Design review of the part built by this model. Coordinates are the model's own, in mm. Face numbers are marked on the shaded views. A direction names the side the tool comes from. Give positions to 0.01 mm unless a question says otherwise; leave off trailing zeros. Write each loop counter-clockwise with the first axis right and the second up, starting at its lowest first coordinate (ties: lowest second). Pieces come first, ordered by that corner, then holes. Notation, with made-up numbers: M -19,-30.75 L 39,-30.75 A20 cw 39,-1.75 Z; hole C 88,7.5 d5. An arc over 180 degrees is marked long. Answer in a Markdown table with one row per item.
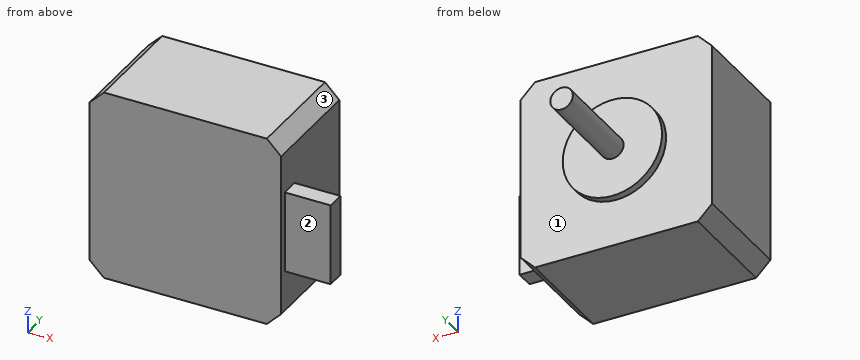
Autodesk Inventor part; units mm, degrees
ref_plane "YZ Plane" through (0, 0, 0) normal (1, 0, 0) x (0, 1, 0)
ref_plane "XZ Plane" through (0, 0, 0) normal (0, 1, 0) x (-1, 0, 0)
ref_plane "XY Plane" through (0, 0, 0) normal (0, 0, 1) x (1, 0, 0)
sketch "Sketch1" plane through (0, 0, 0) normal (0, 1, 0) x (-1, 0, 0)
  line L0 (-18.034, 21.209) -> (18.034, 21.209)
  line L1 (21.209, 18.034) -> (21.209, -18.034)
  line L2 (18.034, -21.209) -> (-18.034, -21.209)
  line L3 (-21.209, -18.034) -> (-21.209, 18.034)
  line L4 (-21.209, 21.209) -> (21.209, -21.209) construction
  line L5 (21.209, 21.209) -> (-21.209, -21.209) construction
  line L6 (21.209, 18.034) -> (18.034, 21.209)
  line L7 (18.034, -21.209) -> (21.209, -18.034)
  line L8 (-18.034, -21.209) -> (-21.209, -18.034)
  line L9 (-21.209, 18.034) -> (-18.034, 21.209)
  point P0 (0, 0)
  dimension "d0" = 42.418
  dimension "d1" = 3.175
  dimension "d2" = 3.175
  dimension "d3" = 3.175
  dimension "d4" = 3.175
  dimension "d5" = 3.175
  dimension "d6" = 3.175
  dimension "d7" = 3.175
  dimension "d8" = 3.175
extrude "Extrusion1" add sketch "Sketch1" along normal blind 23.876
sketch "Sketch2" plane through (0, 23.876, 0) normal (0, 1, 0) x (1, 0, 0)
  circle A0 centre (0, 0) radius 10.9982
  dimension "d11" = 21.9964
extrude "Extrusion2" add sketch "Sketch2" along normal blind 1.651
sketch "Sketch3" plane through (0, 25.527, 0) normal (0, 1, 0) x (1, 0, 0)
  circle A0 centre (0, 0) radius 2.4892
  dimension "d14" = 4.9784
extrude "Extrusion3" add sketch "Sketch3" along normal blind 20.828
sketch "Sketch4" plane through (21.209, 0, 18.034) normal (1, 0, 0) x (0, 0, -1)
  line L0 (9.0162, 1.503) -> (27.0518, 1.503)
  line L1 (27.0518, 1.503) -> (27.0518, 5.5109)
  line L2 (27.0518, 5.5109) -> (9.0162, 5.5109)
  line L3 (9.0162, 5.5109) -> (9.0162, 1.503)
  line L4 (9.0162, 1.503) -> (27.0518, 5.5109) construction
  line L5 (27.0518, 1.503) -> (9.0162, 5.5109) construction
  point P0 (18.034, 0)
  point P1 (18.034, 3.5069)
extrude "Extrusion4" add sketch "Sketch4" along normal blind 10.16
equation "\"d2\" = d1"
equation "\"d3\" = d1"
equation "\"d4\" = d3"
equation "\"d5\" = d1"
equation "\"d6\" = d5"
equation "\"d7\" = d1"
equation "\"d8\" = d7"
properties part number "stepper_17HS4023"
1) Add section A-A (y = 16). Write out the cut boundary in (x, z), and give its area (3 significant figures).
Geometry says:
| item | result |
|---|---|
| outline | M -21.21,-18.03 L -18.03,-21.21 L 18.03,-21.21 L 21.21,-18.03 L 21.21,18.03 L 18.03,21.21 L -18.03,21.21 L -21.21,18.03 Z |
| area | 1,780 mm^2 |
2) To check wall thickness, follow probe 1 along Y at (x, z) = (12.5, -2.5); probe 2 along Y at (x, z) = (4, 2); probe 3 along X at (y, z) = (13, -7.5). State the ranges of each line that lie inside material, in increasing order. Write a range as [from, to].
Geometry says:
| item | result |
|---|---|
| probe 1 | [0, 23.88] |
| probe 2 | [0, 25.53] |
| probe 3 | [-21.21, 21.21] |
3) Insertion check: P1, Ø1.2, axis at x = 26.5, y = 2.5, coming from the +Z side; P2, Ø3, axis at x = 24.5, z = -4, coming from the -Y side; P3, Ø3, axis at x = 26.5, y = 4, coming from the -Z side. Each pin has a flat end and moves straight along its axis. Give the tip position at first contact, or say it passes through.
Geometry says:
| item | result |
|---|---|
| P1 | z = 9.02 |
| P2 | y = 1.5 |
| P3 | z = -9.02 |
4) For the marked faces 1, 2 and 3, list the 3-axis set-ups (+Z, -Z, +X, -X, +Y, -Y) from which the entire face can be reached by the end or side of a thin tool; tool diameter is ignored.
Geometry says:
| item | result |
|---|---|
| face 1 | +Y |
| face 2 | +Z, -Z, +X, -Y |
| face 3 | +Z, +X, +Y, -Y |
5) Add section B-B (z = 0). Write out the cut boundary in (x, y) (3 decimals), and give its area (3 significant figures).
Geometry says:
| item | result |
|---|---|
| outline | M -21.209,0 L 21.209,0 L 21.209,1.503 L 31.369,1.503 L 31.369,5.511 L 21.209,5.511 L 21.209,23.876 L 10.998,23.876 L 10.998,25.527 L 2.489,25.527 L 2.489,46.355 L -2.489,46.355 L -2.489,25.527 L -10.998,25.527 L -10.998,23.876 L -21.209,23.876 Z |
| area | 1,190 mm^2 |
6) Add section C-C (x = 0). Write out the cut boundary in (y, z) (3 decimals).
Geometry says:
| item | result |
|---|---|
| outline | M 0,-21.209 L 23.876,-21.209 L 23.876,-10.998 L 25.527,-10.998 L 25.527,-2.489 L 46.355,-2.489 L 46.355,2.489 L 25.527,2.489 L 25.527,10.998 L 23.876,10.998 L 23.876,21.209 L 0,21.209 Z |
7) Add section D-D (x = -10). Write out the cut boundary in (y, z).
Geometry says:
| item | result |
|---|---|
| outline | M 0,-21.21 L 23.88,-21.21 L 23.88,-4.58 L 25.53,-4.58 L 25.53,4.58 L 23.88,4.58 L 23.88,21.21 L 0,21.21 Z |
